from build123d import *

# Parameters (mm, degrees)
F0_R     = 4.445
F0_R_2   = 2.667
F1_DEPTH = 6.35
F0_R_3   = 1.524
F2_DEPTH = 1.5875
F3_R     = 1.5875


with BuildPart() as f1:
    # F0 (on Top) → F1 (new body)
    with BuildSketch(Plane.XY):
        Circle(F0_R)
        Circle(F0_R_2, mode=Mode.SUBTRACT)
    extrude(amount=F1_DEPTH)

    # F0 (on Top) → F2 (join)
    with BuildSketch(Plane.XY):
        Circle(F0_R_2)
        Circle(F0_R_3, mode=Mode.SUBTRACT)
    extrude(amount=F2_DEPTH)

    # F3
    f3_edges = [f1.edges().sort_by_distance(p)[0] for p in [
        (-4.445, 0, 6.35),
    ]]
    fillet(f3_edges, radius=F3_R)


solid = f1.part
Here's how the part is built. I have some questions about the finished solid (model axes, mm). Coordinates: 2 decimals unless noted, no trailing zeros. Order: outer loops, then holes, each group sorted by start corner. A loop starts at its lowest first (then second) coordinate and runs counter-clockwise, first axis right, second up.
Item 1: I need wall thicknesses on line 1 (Y direction, x = 0, z = 4.2) (3 decimals); line 2 (Y direction, x = 0, z = 0.9) (3 decimals); line 3 (Z direction, x = -0.75, y = -1.75). Which ranges of each line are inside material? Lowest first, please.
Result sheet:
line 1: y = -4.445 to -2.667, 2.667 to 4.445
line 2: y = -4.445 to -1.524, 1.524 to 4.445
line 3: z = 0 to 1.59
Item 2: If we section it at D-D on z = 0.75: List the corners of the cut face in (x, y) for me (3 decimals), plus the area to 3 significant figures.
Result sheet:
outline: circle Ø8.89 at (0, 0); hole circle Ø3.048 at (0, 0)
area: 54.8 mm2
Item 3: If we section it at C-C on z = 2.5: List the corners of the cut face in (x, y) for me (3 decimals).
Result sheet:
outline: circle Ø8.89 at (0, 0); hole circle Ø5.334 at (0, 0)
Item 4: If we mould it in two halves opening along X, with no side actions, what happens to faces 1 (the face through (-0.2, 1.51, 0.78)), 2 (the face through (-0.96, -4.34, 2.35)), 3 (the face through (0, -2, 0))? For each: +X half, -X half, draft (parallel to the pull), parting line (faces both ways), or undercut.
Result sheet:
face 1: undercut
face 2: parting line
face 3: draft
Item 5: For P1, Ø1.8, axis at x = 0, y = 0, coming from the -Z side; P2, Ø3, axis at y = -3.5, z = 3.5, coming from the -X side, each with a flat end and sliding along its axis, tell me the tip position at first contact or that it passes through.
Result sheet:
P1: passes through
P2: stops at x = -3.97
